Part model, mm, in its own coordinate system. A direction names the side the tool comes from. Round coordinates to 2 decimals unless told otherwise and drop trailing zeros. Order: outer loops, then holes, each group sorted by start corner. A loop starts at its lowest first (then second) coordinate and runs counter-clockwise, first axis right, second up. Notation, with made-up numbers: (-37, 1) -> (-18, 1) arc R17 ccw to (-18, 29) -> close; hole circle Ø7 at (0, 28.5). An arc over 180 degrees is marked (long way). Return JSON: item names as keys, results as strings. Group by question number.
from build123d import *

# Parameters (mm, degrees)
CYLINDER_R        = 12
CYLINDER_DEPTH    = 6
CYLINDER001_R     = 9
CYLINDER001_DEPTH = 16


with BuildPart() as cylinder:
    # Cylinder → Cylinder (new body)
    with BuildSketch(Plane.XY):
        Circle(CYLINDER_R)
    extrude(amount=CYLINDER_DEPTH)


with BuildPart() as fusion:
    # Cylinder001 → Cylinder001 (new body)
    with BuildSketch(Plane.XY):
        Circle(CYLINDER001_R)
    extrude(amount=CYLINDER001_DEPTH)

    # Fusion: union Cylinder
    add(cylinder.part)


solid = fusion.part
(1) Probe L1, parallel to Z at x = -2.5, y = 11.25; L2, parallel to X at y = -3.75, z = 15; L3, parallel to Y at x = 2.25, z = 9.5. List the from-to ranges inside material, lowest first. Write a range as [from, to].
(2) Pin check, flat tips, straight feed: P1, Ø1, axis at y = 1, z = 11, coming from the +X side; P2, Ø1.5, axis at y = 8, z = 2, coming from the -X side; P3, Ø6, axis at x = -9, z = 11, coming from the -Y side; P4, Ø4, axis at x = -9, y = -4, coming from the +Z side. Stop position of each tip, or through.
(3) Saw through at C-C, the plane z = 15. List the corners of the cut face in (x, y).
(4) Saw through at A-A, the plane x = 0. List the corners of the cut face in (y, z), and give its area (3 significant figures).
(5) Saw through at D-D, the plane z = 3.75. List the corners of the cut face in (x, y).
(6) Tool access for faces 1 (the flat face through (0, 0, 0)), 2 (the cylindrical face through (-1.172, 8.923, 10.93)): list every direction of +Z, -Z, +X, -X, +Y, -Y with a clear straight run to the whole face (end or side of a thin tool).
Results are:
{
 "1": {"L1": "z = [0, 6]", "L2": "x = [-8.18, 8.18]", "L3": "y = [-8.71, 8.71]"},
 "2": {"P1": "stops at x = 8.99", "P2": "stops at x = -9.56", "P3": "stops at y = -6.71", "P4": "stops at z = 16"},
 "3": {"outline": "circle Ø18 at (0, 0)"},
 "4": {"outline": "(-12, 0) -> (12, 0) -> (12, 6) -> (9, 6) -> (9, 16) -> (-9, 16) -> (-9, 6) -> (-12, 6) -> close", "area": "324 mm^2"},
 "5": {"outline": "circle Ø24 at (0, 0)"},
 "6": {"face 1": "-Z, +X, -X, +Y, -Y", "face 2": "+Z"}
}
